Build history of the part. All positions in model axes, mm. Give positions to 0.01 mm unless a question says otherwise; leave off trailing zeros. Loops run counter-clockwise (first coordinate to the right, second up) from the corner with the lowest first, then second, coordinate; pieces in that order, holes last. Notation, with made-up numbers: M 35.5,73.25 L 81.5,73.25 A20 ccw 81.5,91.25 Z; hole C 67,-10.75 d2. An arc over 180 degrees is marked long. Answer as a JSON object with one key per item and string values. Group by question number.
1. Drill centre lines: line 1 along Z through (x, y) = (-154, -131); line 2 along Z through (x, y) = (-170.5, -128.95); line 3 along Z through (x, y) = (-105, -129.1). Where is each one in solid material? Low to high. Write a range as [from, to].
2. Drop flat-ended pins along their axis: pin 1 Ø0.8 at (y, z) = (-129.5, -114.5) entering from -X; pin 2 Ø1.3 at (x, y) = (-178, -130) entering from +Z; pin 3 Ø0.8 at (x, y) = (-75, -130.5) entering from -Z. Give the stop position or say it passes through.
3. Slice it at D-D (x = -175). Give the number of separate pieces and of enclosed holes in the cut face, then the cut area to 3 significant figures.
4. Slice it at B-B (x = -163). List the corners of the cut face in (y, z), then the cut area to 3 significant figures.
5. Slice it at C-C (x = -130.5). List the corners of the cut face in (y, z), then the cut area to 3 significant figures.
6. Slice it at A-A (x = -148). List the corners of the cut face in (y, z).
from build123d import *

# Parameters (mm, degrees)
SKETCH1_W           = 119.784208154
SKETCH1_H           = 2.7
BOSS_EXTRUDE1_DEPTH = 80
BOSS_EXTRUDE2_DEPTH = 2.7


with BuildPart() as part:
    # Sketch1 → Boss-Extrude1 (new, symmetric)
    with BuildSketch(Plane.XY):
        with Locations((-129.502935336, -130)):
            Rectangle(SKETCH1_W, SKETCH1_H)
    extrude(amount=BOSS_EXTRUDE1_DEPTH, both=True)

    # Sketch2 → Boss-Extrude2 (add)
    with BuildSketch(Plane(origin=(0, -128.65, 0), x_dir=(1, 0, 0), z_dir=(0, 1, 0))):
        with BuildLine():
            Line((-169.648055861, -113.2), (-93.105798555, -113.2))
            add(Edge.make_bspline(
                [(-81.948677427, -80), (-86.342810108, -90.98944534), (-84.004205112, -103.888102009), (-93.105798555, -113.2)],
                knots=[0, 0, 0, 0, 1, 1, 1, 1], degree=3))
            Line((-81.948677427, -80), (-81.948677427, -77.720195576))
            Line((-81.948677427, -77.720195576), (-177.731759246, -77.720195576))
            Line((-177.731759246, -77.720195576), (-177.731759246, -80))
            Line((-177.731759246, -80), (-144.395039413, -80))
            Line((-144.395039413, -80), (-144.395039413, -85))
            Line((-144.395039413, -85), (-177.731759246, -85))
            Line((-177.731759246, -85), (-177.731759246, -95.646483093))
            add(Edge.make_bspline(
                [(-169.648055861, -105.087652523), (-167.760228738, -94.514197341), (-177.731759246, -95.646483093)],
                knots=[0, 0, 0, 1, 1, 1], degree=2))
            Line((-169.648055861, -105.087652523), (-169.648055861, -113.2))
        make_face()
        with BuildLine():
            Line((-177.731759246, 80), (-177.731759246, 77.720195576))
            Line((-177.731759246, 77.720195576), (-81.948677427, 77.720195576))
            Line((-81.948677427, 77.720195576), (-81.948677427, 80))
            add(Edge.make_bspline(
                [(-81.948677427, 80), (-86.342810108, 90.98944534), (-84.004205112, 103.888102009), (-93.105798555, 113.2)],
                knots=[0, 0, 0, 0, 1, 1, 1, 1], degree=3))
            Line((-93.105798555, 113.2), (-97.105798555, 113.2))
            Line((-97.105798555, 113.2), (-97.105798555, 118.2))
            Line((-97.105798555, 118.2), (-112.105798555, 118.2))
            Line((-112.105798555, 118.2), (-112.105798555, 113.2))
            Line((-112.105798555, 113.2), (-127.105798555, 113.2))
            Line((-127.105798555, 113.2), (-127.105798555, 118.2))
            Line((-127.105798555, 118.2), (-142.105798555, 118.2))
            Line((-142.105798555, 118.2), (-142.105798555, 113.2))
            Line((-142.105798555, 113.2), (-153.105798555, 113.2))
            add(Edge.make_bspline(
                [(-153.105798555, 113.2), (-158.310437451, 123.519674565), (-159.620228805, 135)],
                knots=[0, 0, 0, 1, 1, 1], degree=2))
            Line((-159.620228805, 135), (-159.620228805, 140))
            Line((-159.620228805, 140), (-169.620228805, 140))
            Line((-169.620228805, 140), (-169.620228805, 135))
            Line((-169.620228805, 135), (-177.731759246, 135))
            Line((-177.731759246, 135), (-177.731759246, 118.728473066))
            add(Edge.make_bspline(
                [(-177.731759246, 93.702985707), (-160.836478184, 106.395581303), (-177.731759246, 118.728473066)],
                knots=[0, 0, 0, 1, 1, 1], degree=2))
            Line((-177.731759246, 93.702985707), (-177.731759246, 85))
            Line((-177.731759246, 85), (-144.395039413, 85))
            Line((-144.395039413, 85), (-144.395039413, 80))
            Line((-144.395039413, 80), (-177.731759246, 80))
        make_face()
    extrude(amount=-BOSS_EXTRUDE2_DEPTH)


solid = part.part
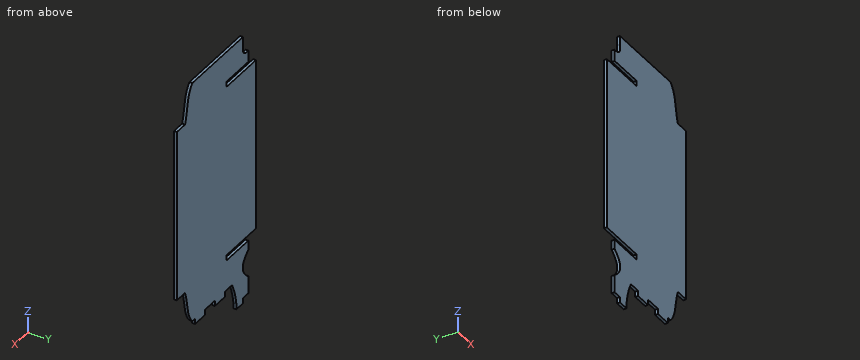
Established:
{
 "1": {"line 1": "z = [-115.04, -85], [-80, 80], [85, 113.2]", "line 2": "z = [-135, -111.04], [-101.55, -85], [-80, 80], [85, 97.73]", "line 3": "z = [-118.2, 113.2]"},
 "2": {"pin 1": "stops at x = -173.31", "pin 2": "stops at z = 95.65", "pin 3": "stops at z = -80"},
 "3": {"separate pieces": "4", "enclosed holes": "0", "area": "540 mm^2"},
 "4": {"outline": "M -131.35,-140 L -128.65,-140 L -128.65,-85 L -131.35,-85 Z; M -131.35,-80 L -128.65,-80 L -128.65,80 L -131.35,80 Z; M -131.35,85 L -128.65,85 L -128.65,113.2 L -131.35,113.2 Z", "area": "657 mm^2"},
 "5": {"outline": "M -131.35,-118.2 L -128.65,-118.2 L -128.65,113.2 L -131.35,113.2 Z", "area": "625 mm^2"},
 "6": {"outline": "M -131.35,-113.2 L -128.65,-113.2 L -128.65,-85 L -131.35,-85 Z; M -131.35,-80 L -128.65,-80 L -128.65,80 L -131.35,80 Z; M -131.35,85 L -128.65,85 L -128.65,113.2 L -131.35,113.2 Z"}
}
